Here's the drawing with two shaded views (mm, measured from the low corner). I have some questions. A direction names the side the tool comes from. Coordinates: 2 decimals unless noted, no trailing zeros. Loops run counter-clockwise (first coordinate to the right, second up) from the corner with the lowest first, then second, coordinate; pieces in that order, holes last. Notation, with made-up numbers: (-28.5, -11) - (11.5, -11) arc R11 ccw to (11.5, 1) - close; hole circle Ø9 at (7.25, -13). An arc over 180 degrees is marked (long way). Use a Markdown table: item, result.
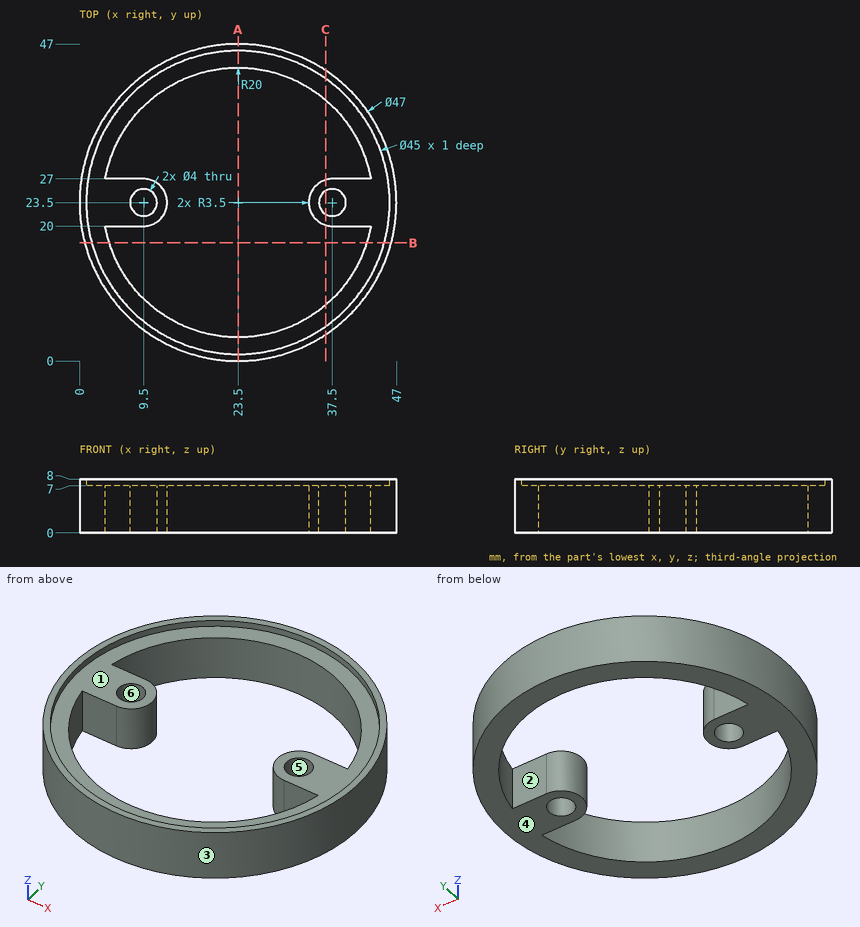
Q1. Which directions (+Z, -Z, +X, -X, +Y, -Y) give clear straight access to the entire face, cutting with the end or side of a thin tool? Please do the marked faces 1 and 2.
Check values:
| item | result |
|---|---|
| face 1 | +Z |
| face 2 | +Z, -Z |
Q2. Please list where these lines run through material, in increasing order: L1, parallel to Y at x = 23.5, z = 7.4; L2, parallel to Y at x = 5, z = 3.25; L3, parallel to Y at x = 37.5, z = 4. Write a range as from..to.
Check values:
| item | result |
|---|---|
| L1 | 0..1, 46..47 |
| L2 | 9.01..15.9, 20..27, 31.1..37.99 |
| L3 | 4.63..9.22, 20..21.5, 25.5..27, 37.78..42.37 |
Q3. Will these pins go through, and if not, where does the flat tip stop? P1, Ø2, axis at y = 29, z = 3.5, coming from the -X side; P2, Ø1.7, axis at x = 7, z = 4.5, coming from the -Y side; P3, Ø4.5, axis at x = 39.5, z = 3.5, coming from the +Y side.
Check values:
| item | result |
|---|---|
| P1 | x = 0.43 |
| P2 | y = 5.97 |
| P3 | y = 42.56 |
Q4. I want a section at A-A, the plane x = 23.5. Write out the boundary of the cut face in (y, z).
Check values:
| item | result |
|---|---|
| outline | (0, 0) - (3.5, 0) - (3.5, 7) - (1, 7) - (1, 8) - (0, 8) - close; (43.5, 0) - (47, 0) - (47, 8) - (46, 8) - (46, 7) - (43.5, 7) - close |
Q5. I want a section at C-C, the plane x = 36.5. Write out the boundary of the cut face in (y, z).
Check values:
| item | result |
|---|---|
| outline | (3.92, 0) - (8.3, 0) - (8.3, 7) - (5.14, 7) - (5.14, 8) - (3.92, 8) - close; (20.15, 0) - (21.77, 0) - (21.77, 7) - (20.15, 7) - close; (25.23, 0) - (26.85, 0) - (26.85, 7) - (25.23, 7) - close; (38.7, 0) - (43.08, 0) - (43.08, 8) - (41.86, 8) - (41.86, 7) - (38.7, 7) - close |
Q6. I want a section at B-B, the plane y = 17.5. Write out the boundary of the cut face in (x, z), then the cut area to 3 significant figures.
Check values:
| item | result |
|---|---|
| outline | (0.78, 0) - (4.42, 0) - (4.42, 7) - (1.81, 7) - (1.81, 8) - (0.78, 8) - close; (42.58, 0) - (46.22, 0) - (46.22, 8) - (45.19, 8) - (45.19, 7) - (42.58, 7) - close |
| area | 53.1 mm^2 |
Q7. If we mould it in two halves opening along X, with no side actions, what happens to the marked faces 3, 4, 5 and 6? For each: pulls with the +X half, pulls with the -X half, needs draft (parallel to the pull), parting line crosses it, or undercut.
Check values:
| item | result |
|---|---|
| face 3 | parting line crosses it |
| face 4 | needs draft |
| face 5 | undercut |
| face 6 | undercut |
